Could you check a few things on this model? Use its own coordinates, in mm. A direction names the side the tool comes from. Give positions to 0.01 mm unless a question says otherwise; leave off trailing zeros. Loops run counter-clockwise (first coordinate to the right, second up) from the corner with the lowest first, then second, coordinate; pieces in that order, holes last. Notation, with made-up numbers: (60, 4.5) - (73, 4.5) arc R32 ccw to (73, 38.5) - close; hole circle Ø1 at (36, 56). An arc over 180 degrees is marked (long way). Write each question's results on one line, items separated by ' | '. Start each with the question number.
Autodesk Inventor part; units mm, degrees
ref_plane "YZ Plane" through (0, 0, 0) normal (1, 0, 0) x (0, 1, 0)
ref_plane "XZ Plane" through (0, 0, 0) normal (0, 1, 0) x (-1, 0, 0)
ref_plane "XY Plane" through (0, 0, 0) normal (0, 0, 1) x (1, 0, 0)
sketch "Náčrt1" plane through (0, 0, 0) normal (0, 0, 1) x (1, 0, 0)
  line L0 (13.97, 23.865) -> (13.97, 9.144)
  line L1 (0, 9.144) -> (0, 0)
  line L2 (4.5409, 9.144) -> (0, 9.144)
  line L3 (4.5409, 8.255) -> (4.5409, 9.144)
  line L4 (3.2709, 6.985) -> (4.5409, 8.255)
  line L5 (3.2709, 4.318) -> (3.2709, 6.985)
  line L6 (8.7319, 9.144) -> (8.7319, 8.255)
  line L7 (13.97, 9.144) -> (8.7319, 9.144)
  line L8 (8.7319, 8.255) -> (10.0019, 6.985)
  line L9 (10.0019, 6.985) -> (10.0019, 4.318)
  line L10 (10.0019, 4.318) -> (3.2709, 4.318)
  line L11 (0, 0) -> (19.97, 0)
  line L12 (13.97, 22.5956) -> (13.97, 25.1349)
  line L13 (13.97, 20.4353) -> (13.97, 18.035)
  line L14 (13.97, 25.1349) -> (19.97, 25.1349)
  line L15 (19.97, 25.1349) -> (19.97, 0)
extrude "Vysunutí1" add sketch "Náčrt1" against normal blind 32.6
sketch "Náčrt2" plane through (19.97, 0, 0) normal (1, 0, 0) x (0, 0, -1)
  line L0 (0, 25.1349) -> (32.6, 25.1349)
  line L1 (16.3, 25.1349) -> (4.746, 25.1349)
  line L2 (4.746, 25.1349) -> (4.746, 12.9539)
  line L3 (16.3, 25.1349) -> (27.854, 25.1349)
  line L4 (27.854, 25.1349) -> (27.854, 12.9539)
  line L5 (27.854, 12.9539) -> (4.746, 12.9539)
  circle A0 centre (2.8, 19.2349) radius 1.2
  line L6 (16.3, 25.1349) -> (16.3, 15.9225)
  circle A1 centre (29.8, 19.2349) radius 1.2
  point P0 (0, 0)
  point P1 (4.746, 19.0444)
  dimension "d2" = 11.554
  dimension "d3" = 12.181
  dimension "d4" = 11.554
  dimension "d7" = 2.4
  dimension "d8" = 5.9
  dimension "d9" = 1.946
extrude "Vysunutí2" cut sketch "Náčrt2" against normal blind 32.6 contours L0 L4 L5 L2
extrude "Vysunutí3" cut sketch "Náčrt2" against normal blind 32.6 contours A0 | A1
fillet "Zaoblení1" radius 2 4 edges at (16.97, 25.1349, 0) (16.97, 25.1349, -4.746) (16.97, 25.1349, -27.854) (16.97, 25.1349, -32.6)
sketch "Náčrt3" plane through (0, 0, 0) normal (0, -1, 0) x (1, 0, 0)
  point P0 (0, 0)
sketch "Náčrt8" plane through (0, 0, 0) normal (-1, 0, 0) x (0, 0, 1)
  line L0 (0, 9.144) -> (-32.6, 9.144)
  line L1 (0, 0) -> (-32.6, 0)
  circle A0 centre (-16.3, 17.144) radius 2.25
  line L2 (-23.3, 9.144) -> (-9.3, 9.144)
  line L3 (-9.3, 9.144) -> (-9.3, 23.144)
  line L4 (-9.3, 23.144) -> (-23.3, 23.144)
  line L5 (-23.3, 23.144) -> (-23.3, 9.144)
  line L6 (0, 9.144) -> (0, 0)
  line L7 (0, 9.144) -> (0, 0)
  line L8 (0, 4.572) -> (9.3918, 4.572)
  circle A1 centre (-16.3, -8) radius 2.25
  line L9 (-23.3, 0) -> (-9.3, 0)
  line L10 (-9.3, 0) -> (-9.3, -14)
  line L11 (-9.3, -14) -> (-23.3, -14)
  line L12 (-23.3, -14) -> (-23.3, 0)
  point P0 (-16.3, 9.144)
  point P1 (-16.3, 9.144)
  point P2 (-16.3, 0)
  point P3 (-16.3, 0)
  dimension "d35" = 4.5
  dimension "d36" = 8
  dimension "k" = 14
  dimension "d42" = 14
  dimension "d43" = 7
  dimension "d44" = 7
extrude "Vysunutí7" add sketch "Náčrt8" against normal up to surface (3.2709 mm away)
fillet "Zaoblení2" radius 2 4 edges at (1.6355, 9.144, -9.3) (1.6355, 0, -9.3) (1.6355, 9.144, -23.3) (1.6355, 0, -23.3)
equation "\"d43\" = 0.5 * k"
properties part number "Motor_holder_double" material "Měď"
Q1. I want a section at D-D, the plane x = 16. List the corners of the cut face in (y, z) for me, then the cut area to 3 significant figures.
Q2. I want a section at C-C, the plane z = -3.5. List the corners of the cut face in (x, y) for me (3 decimals).
Q3. I need wall thicknesses on L1, parallel to Y at x = 15.35, z = -2.8; L2, parallel to X at y = 10, z = -22; L3, parallel to Y at x = 18.5, z = -15. Which ranges of each line are inside material? Lowest first, please. Write a range as from..to.
Q4. If we mould it in two halves opening along Z, with no side actions, what happens to faces 5 (the face through (17.012, 24.533, -32.03)), 6 (the face through (14.3, 9.2, 0)), 7 (the face through (17, 12.954, -16)), 8 (the face through (4.541, 8.7, -16.1))? For each: +Z half, -Z half, draft (parallel to the pull), parting line (faces both ways), or undercut.
Q5. Which directions (+Z, -Z, +X, -X, +Y, -Y) give clear straight access to the entire face, cutting with the end or side of a thin tool? Please do faces 1 (the face through (10.002, 6, -16)), 2 (the face through (17, 18, -27.854)), 3 (the face through (2, -8, -23.3)), 4 (the face through (3.271, -5, -16)).
Q6. I want a section at B-B, the plane z = -16.3. List the corners of the cut face in (x, y) for me (3 decimals), then the cut area to 3 significant figures.
Q7. I'm going to push flat-ended pins straight in: pin 1 Ø3 at (x, z) = (15.5, -5.5) entering from +Y; pin 2 Ø2 at (x, z) = (16, -21) entering from -Y; pin 3 Ø2 at (x, z) = (8, -16.5) entering from +Y; pin 4 Ø5 at (x, y) = (10, 19.5) entering from +Z. Where does each tip first touch, or does it pass through?
Q8. I want a section at A-A, the plane y = -8. List the corners of the cut face in (x, z) for me, then the cut area to 3 significant figures.
Conclusion:
1) outline: (0, -32.6) - (23.13, -32.6) arc R2 ccw to (25.13, -30.6) - (25.13, -29.85) arc R2 ccw to (23.13, -27.85) - (12.95, -27.85) - (12.95, -4.75) - (23.13, -4.75) arc R2 ccw to (25.13, -2.75) - (25.13, -2) arc R2 ccw to (23.13, 0) - (0, 0) - close; hole circle Ø2.4 at (19.23, -29.8); hole circle Ø2.4 at (19.23, -2.8) | area: 525 mm^2
2) outline: (0, 0) - (19.97, 0) - (19.97, 18.26) - (13.97, 18.26) - (13.97, 9.144) - (8.732, 9.144) - (8.732, 8.255) - (10.002, 6.985) - (10.002, 4.318) - (3.271, 4.318) - (3.271, 6.985) - (4.541, 8.255) - (4.541, 9.144) - (0, 9.144) - close; (13.97, 20.21) - (19.97, 20.21) - (19.97, 24.987) - (13.97, 24.987) - close
3) L1: 0..18.03, 20.43..25.13 | L2: 0..3.27, 13.97..19.97 | L3: 0..12.95
4) face 5: -Z half | face 6: +Z half | face 7: undercut | face 8: draft
5) face 1: +Z, -Z | face 2: +X, -X, +Y | face 3: -Z, +X, -X, -Y | face 4: +Z, -Z, +X, -Y
6) outline: (0, -14) - (3.271, -14) - (3.271, -10.25) - (0, -10.25) - close; (0, -5.75) - (3.271, -5.75) - (3.271, 0) - (19.97, 0) - (19.97, 12.954) - (13.97, 12.954) - (13.97, 9.144) - (8.732, 9.144) - (8.732, 8.255) - (10.002, 6.985) - (10.002, 4.318) - (3.271, 4.318) - (3.271, 6.985) - (4.541, 8.255) - (4.541, 9.144) - (3.271, 9.144) - (3.271, 14.894) - (0, 14.894) - close; (0, 19.394) - (3.271, 19.394) - (3.271, 23.144) - (0, 23.144) - close | area: 239 mm^2
7) pin 1: y = 24.69 | pin 2: y = 0 | pin 3: y = 9.14 | pin 4: through
8) outline: (0, -23.3) - (3.27, -23.3) - (3.27, -18.55) - (0, -18.55) - close; (0, -14.05) - (3.27, -14.05) - (3.27, -9.3) - (0, -9.3) - close | area: 31.1 mm^2
